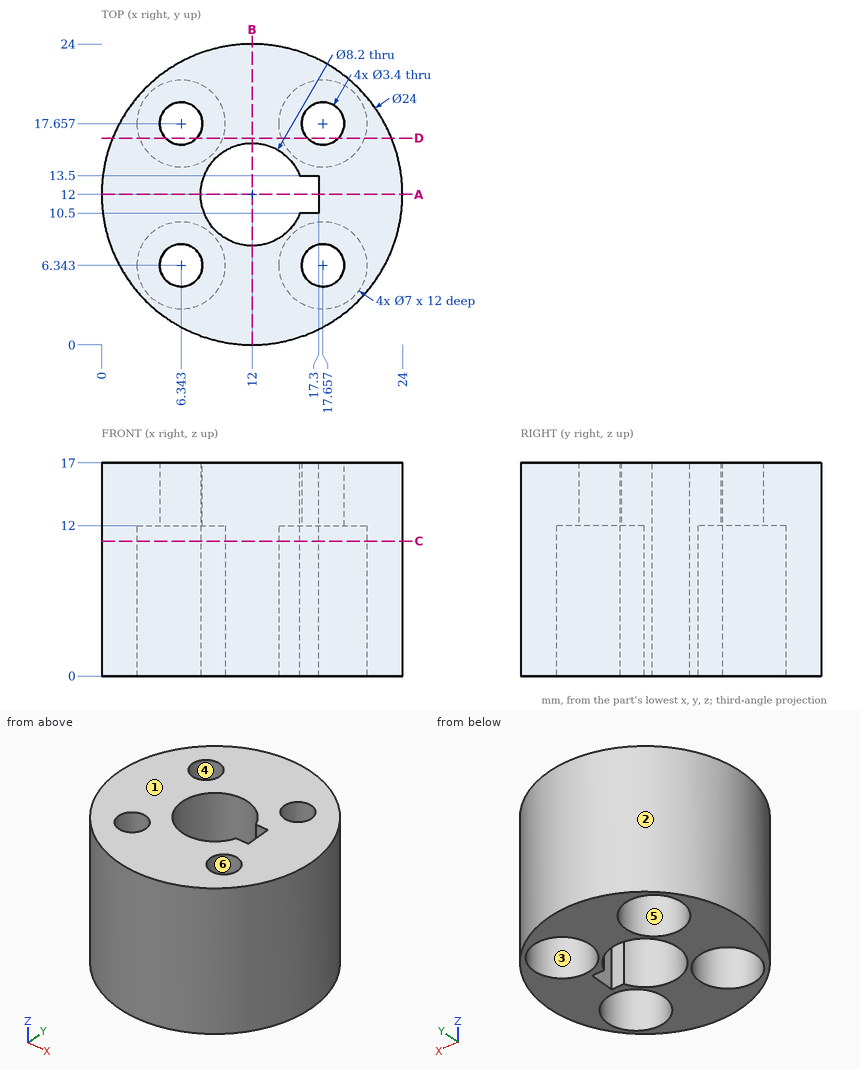
The drawing under review shows one solid part. Ordinate dimensions are in mm from its lowest x, y, z. A direction names the side the tool comes from. Coordinates: 2 decimals unless noted, no trailing zeros. Write each loop counter-clockwise with the first axis right and the second up, starting at its lowest first coordinate (ties: lowest second). Pieces come first, ordered by that corner, then holes.
1) Machinability: for the marked faces 5 and 6, which of the approach directions +Z, -Z, +X, -X, +Y, -Y give a long, thin tool a straight path to every point of the face, cutting with its end or side? Answer none if there is none.
2) To check wall thickness, follow L1, parallel to Y at x = 19.5, z = 1.5; L2, parallel to Y at x = 19.75, z = 11. State the ranges of each line that lie inside material, in increasing order.
3) Insertion check: pin 1 (1.2 mm diameter, centred on x = 16.5, z = 8, fed in from +Y); pin 2 (2 mm diameter, centred on x = 5, z = 2.5, fed in from -Y); pin 3 (4.5 mm diameter, centred on x = 17.66, y = 6.34, fed in from +Z); pin 4 (2 mm diameter, centred on x = 4.5, z = 14.5, fed in from -Y). Each pin has a flat end and moves straight along its axis. Give the tip position at first contact, or say it passes through.
4) Mouldability with a two-part tool opening along Y and no side actions: class the marked faces 1, 2, 3 and 4 as +Y half, -Y half, draft (parallel to the pull), parting line (faces both ways), or undercut.
5) Add section B-B (x = 12). Write out the cut boundary in (y, z), plus the area to 3 significant figures.
6) Add section A-A (y = 12). Write out the cut boundary in (x, z).
7) Add section C-C (z = 10.75). Write out the cut boundary in (x, y), plus the area to 3 significant figures.
8) Add section D-D (y = 16.5). Write out the cut boundary in (x, z).
Check result:
1. face 5: -Z
1. face 6: +Z, -Z
2. L1: y = 2.63 to 3.37, 9.32 to 14.68, 20.63 to 21.37
2. L2: y = 2.84 to 3.54, 9.15 to 14.85, 20.46 to 21.16
3. pin 1: stops at y = 23.35
3. pin 2: stops at y = 1.61
3. pin 3: stops at z = 17
3. pin 4: stops at y = 1.91
4. face 1: draft
4. face 2: parting line
4. face 3: undercut
4. face 4: undercut
5. outline: (0, 0) - (7.9, 0) - (7.9, 17) - (0, 17) - close; (16.1, 0) - (24, 0) - (24, 17) - (16.1, 17) - close
5. area: 269 mm2
6. outline: (0, 0) - (7.9, 0) - (7.9, 17) - (0, 17) - close; (17.3, 0) - (24, 0) - (24, 17) - (17.3, 17) - close
7. outline: circle Ø24 at (12, 12); hole circle Ø7 at (6.34, 6.34); hole circle Ø7 at (6.34, 17.66); hole circle Ø7 at (17.66, 6.34); hole circle Ø7 at (17.66, 17.66); hole (15.82, 10.5) - (17.3, 10.5) - (17.3, 13.5) - (15.82, 13.5) arc R4.1 ccw (long way) to start
7. area: 242 mm2
8. outline: (0.88, 0) - (3.04, 0) - (3.04, 12) - (5.1, 12) - (5.1, 17) - (0.88, 17) - close; (7.59, 12) - (9.65, 12) - (9.65, 0) - (14.35, 0) - (14.35, 12) - (16.41, 12) - (16.41, 17) - (7.59, 17) - close; (18.9, 12) - (20.96, 12) - (20.96, 0) - (23.12, 0) - (23.12, 17) - (18.9, 17) - close
